The drawing under review shows one solid part. Ordinate dimensions are in mm from its lowest x, y, z. Give positions to 0.01 mm unless a question says otherwise; leave off trailing zeros. Order: outer loops, then holes, each group sorted by start corner. A loop starts at its lowest first (then second) coordinate and runs counter-clockwise, first axis right, second up. Notation, with made-up numbers: (-15, -39) -> (36, -39) arc R29 cw to (36, -12) -> close; hole circle Ø11 at (20, 84). An arc over 180 degrees is marked (long way). Use a Markdown table: item, result. Add a question column.
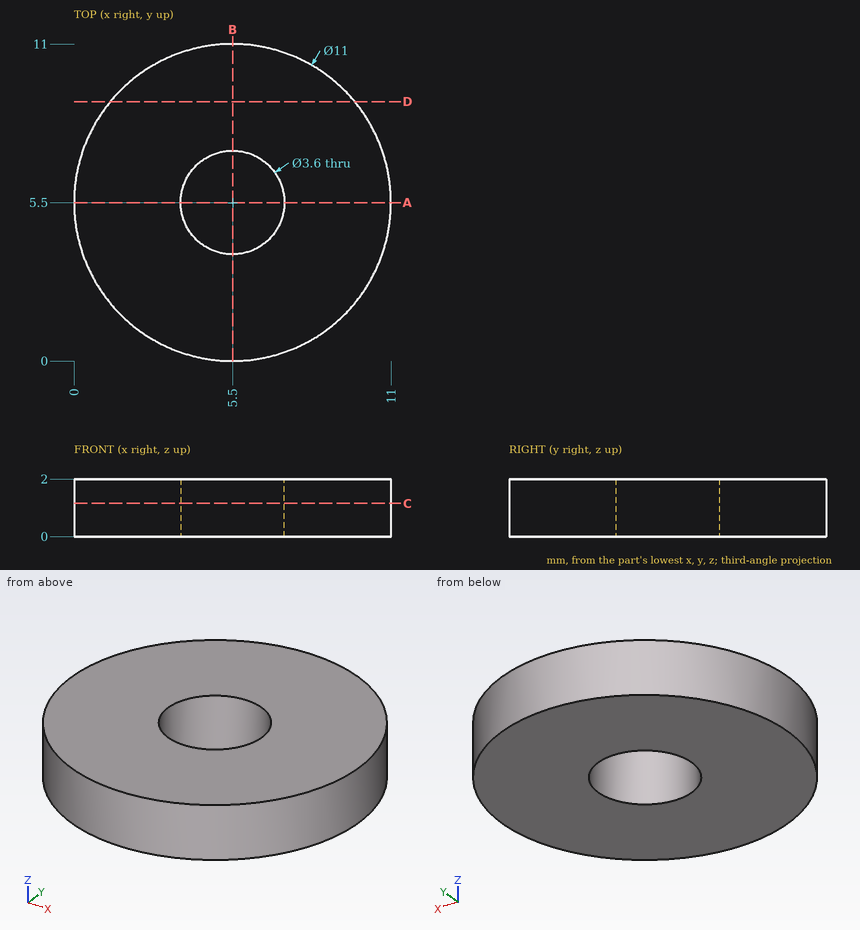
1) Insertion check: pin 1 (3 mm diameter, centred on x = 5.5, y = 5.5, fed in from -Z); pin 2 (1 mm diameter, centred on x = 7, y = 5.5, fed in from -Z). Each pin has a flat end and moves straight along its axis. Give the tip position at first contact, or say it passes through.
2) Add section C-C (z = 1.15). Give the boundary of the cut face in (x, y).
3) For L1, parallel to Y at x = 5.5, z = 1.15; L2, parallel to Y at x = 5, z = 0.75; L3, parallel to Y at x = 8, z = 0.4, list the stretches that pass through material, from the lowest coordinate up. Write a range as [from, to].
4) Add section D-D (y = 9). Give the boundary of the cut face in (x, z).
5) Add section A-A (y = 5.5). Give the boundary of the cut face in (x, z), then the cut area to 3 significant figures.
Worked answers:
| question | item | result |
|---|---|---|
| 1 | pin 1 | through |
| 1 | pin 2 | z = 0 |
| 2 | outline | circle Ø11 at (5.5, 5.5); hole circle Ø3.6 at (5.5, 5.5) |
| 3 | L1 | [0, 3.7], [7.3, 11] |
| 3 | L2 | [0.02, 3.77], [7.23, 10.98] |
| 3 | L3 | [0.6, 10.4] |
| 4 | outline | (1.26, 0) -> (9.74, 0) -> (9.74, 2) -> (1.26, 2) -> close |
| 5 | outline | (0, 0) -> (3.7, 0) -> (3.7, 2) -> (0, 2) -> close; (7.3, 0) -> (11, 0) -> (11, 2) -> (7.3, 2) -> close |
| 5 | area | 14.8 mm^2 |
